Geometry: final body of the model. Coordinates: model frame, mm. A direction names the side the tool comes from. Give positions to 0.01 mm unless a question says otherwise; leave off trailing zeros. Order: outer loops, then holes, each group sorted by start corner. A loop starts at its lowest first (then second) coordinate and runs counter-clockwise, first axis right, second up. Notation, with made-up numbers: (-35.5, 48) -> (17.5, 48) arc R19 ccw to (17.5, 66) -> close; hole circle Ø10 at (83, 24). An arc over 180 degrees is marked (long way). One line per question, with ' | ' between items.
from build123d import *

# Parameters (mm, degrees)
F1_DEPTH  = 2
F3_DEPTH  = 2
F5_DEPTH  = 1
F6_R      = 0.84006
F7_DEPTH  = 1
F8_R      = 0.772284
F9_DEPTH  = 1
F10_W     = 0.575737
F10_H     = 2.122555
F10_W_2   = 0.4
F10_H_2   = 2.778417
F10_H_3   = 2.12387
F10_W_3   = 0.545456
F10_H_4   = 1.760233
F10_W_4   = 0.581819
F10_H_5   = 3.127278
F10_W_5   = 0.472728
F10_H_6   = 4.072734
F10_W_6   = 0.400001
F10_H_7   = 4.181825
F10_W_7   = 0.436365
F10_H_8   = 4.218189
F10_W_8   = 0.509092
F10_H_9   = 3.018187
F10_W_9   = 0.507496
F10_H_10  = 2.769646
F10_W_10  = 0.811112
F11_DEPTH = 0.5


with BuildPart() as f1:
    # F0 (on Top) → F1 (new body)
    with BuildSketch(Plane.XY):
        with BuildLine():
            Line((17.5, 25), (-17.5, 25))
            ThreePointArc((-17.5, 25), (-22.803301, 22.803301), (-25, 17.5))
            Line((-25, 17.5), (-25, -17.5))
            ThreePointArc((-25, -17.5), (-22.803301, -22.803301), (-17.5, -25))
            Line((-17.5, -25), (17.5, -25))
            ThreePointArc((17.5, -25), (22.803301, -22.803301), (25, -17.5))
            Line((25, -17.5), (25, 17.5))
            ThreePointArc((25, 17.5), (22.803301, 22.803301), (17.5, 25))
        make_face()
    extrude(amount=F1_DEPTH)

    # F2 (on face) → F3 (join)
    with BuildSketch(Plane.XY.offset(2)):
        with BuildLine():
            ThreePointArc((-17.337266, -6.77024), (-16.986234, -5.655714), (-16.596286, -4.5542))
            ThreePointArc((-16.596286, -4.5542), (-17.030893, -5.640781), (-17.337266, -6.77024))
        make_face()
        with BuildLine():
            ThreePointArc((0, 13.707489), (-10.053503, 6.171922), (-16.596286, -4.5542))
            ThreePointArc((-16.596286, -4.5542), (-16.986234, -5.655714), (-17.337266, -6.77024))
            ThreePointArc((-17.337266, -6.77024), (-15.200345, -15.343852), (-7.146251, -18.977696))
            ThreePointArc((-7.146251, -18.977696), (2.212472, -19.631089), (11.51198, -18.393445))
            ThreePointArc((11.51198, -18.393445), (18.229392, -13.509449), (18.713062, -5.218303))
            ThreePointArc((18.713062, -5.218303), (18.502407, -4.757976), (18.285647, -4.300492))
            ThreePointArc((18.285647, -4.300492), (10.706603, 6.29139), (0, 13.707489))
        make_face()
        with BuildLine():
            ThreePointArc((18.713062, -5.218303), (18.511326, -4.753823), (18.285647, -4.300492))
            ThreePointArc((18.285647, -4.300492), (18.502407, -4.757976), (18.713062, -5.218303))
        make_face()
    extrude(amount=F3_DEPTH)

    # F4 (on face) → F5 (cut)
    with BuildSketch(Plane.XY.offset(4)):
        with BuildLine():
            Line((-6.871892, 2.191255), (-9.063148, 2.191255))
            ThreePointArc((-9.063148, 2.191255), (-11.253164, 0.073695), (-9.210455, -2.186298))
            Line((-9.210455, -2.186298), (-8.925119, -2.186904))
            Line((-8.925119, -2.186904), (-6.876542, -2.191251))
            ThreePointArc((-6.876542, -2.191251), (-4.680638, -0.002325), (-6.871892, 2.191255))
        make_face()
        with BuildLine():
            Line((-8.925119, -2.186904), (-9.210455, -2.186298))
            ThreePointArc((-9.210455, -2.186298), (-9.067797, -2.191251), (-8.925119, -2.186904))
        make_face()
        with BuildLine():
            Line((10.128108, 2.191255), (7.936852, 2.191255))
            ThreePointArc((7.936852, 2.191255), (5.746836, 0.073695), (7.789545, -2.186298))
            Line((7.789545, -2.186298), (8.074881, -2.186904))
            Line((8.074881, -2.186904), (10.123458, -2.191251))
            ThreePointArc((10.123458, -2.191251), (12.319362, -0.002325), (10.128108, 2.191255))
        make_face()
        with BuildLine():
            Line((8.074881, -2.186904), (7.789545, -2.186298))
            ThreePointArc((7.789545, -2.186298), (7.932203, -2.191251), (8.074881, -2.186904))
        make_face()
        with BuildLine():
            ThreePointArc((-6.770146, -12.095645), (-6.464266, -11.95017), (-6.153883, -11.814569))
            ThreePointArc((-6.153883, -11.814569), (-6.482713, -11.909726), (-6.770146, -12.095645))
        make_face()
        with BuildLine():
            ThreePointArc((4.085766, -12.978509), (-0.882645, -11.0645), (-6.153883, -11.814569))
            ThreePointArc((-6.153883, -11.814569), (-6.464266, -11.95017), (-6.770146, -12.095645))
            ThreePointArc((-6.770146, -12.095645), (-7.094568, -13.392527), (-5.995244, -14.153211))
            ThreePointArc((-5.995244, -14.153211), (-5.884481, -14.14233), (-5.773655, -14.132122))
            ThreePointArc((-5.773655, -14.132122), (-1.437532, -14.261511), (2.746676, -15.40655))
            ThreePointArc((2.746676, -15.40655), (4.494557, -14.787244), (4.085766, -12.978509))
        make_face()
        with BuildLine():
            ThreePointArc((-5.773655, -14.132122), (-5.884481, -14.14233), (-5.995244, -14.153211))
            ThreePointArc((-5.995244, -14.153211), (-5.883949, -14.147927), (-5.773655, -14.132122))
        make_face()
    extrude(amount=-F5_DEPTH, mode=Mode.SUBTRACT)

    # F6 (on face) → F7 (join)
    with BuildSketch(Plane.XY.offset(3)):
        with Locations((-8.223088, 0)):
            Circle(F6_R)
    extrude(amount=F7_DEPTH)

    # F8 (on face) → F9 (join)
    with BuildSketch(Plane.XY.offset(3)):
        with Locations((9.100624, 0)):
            Circle(F8_R)
    extrude(amount=F9_DEPTH)

    # F10 (on face) → F11 (cut)
    with BuildSketch(Plane.XY.offset(4)):
        with Locations((-10.134581, -3.984638)):
            Rectangle(F10_W, F10_H)
        with Locations((-7.127401, -4.31257)):
            Rectangle(F10_W_2, F10_H_2)
        with Locations((-6.472855, -3.985296)):
            Rectangle(F10_W_2, F10_H_3)
        with Locations((-5.818308, -3.803477)):
            Rectangle(F10_W_3, F10_H_4)
        with Locations((7.317732, -4.503073)):
            Rectangle(F10_W_4, F10_H_5)
        with Locations((8.317734, -4.939437)):
            Rectangle(F10_W_5, F10_H_6)
        with Locations((9.263191, -4.957618)):
            Rectangle(F10_W_6, F10_H_7)
        with Locations((10.154101, -4.939436)):
            Rectangle(F10_W_7, F10_H_8)
        with Locations((11.208649, -4.375799)):
            Rectangle(F10_W_8, F10_H_9)
        with Locations((-9.240523, -4.308184)):
            Rectangle(F10_W_9, F10_H_10)
        with Locations((-8.240381, -4.31257)):
            Rectangle(F10_W_10, F10_H_2)
    extrude(amount=-F11_DEPTH, mode=Mode.SUBTRACT)


solid = f1.part
1) Pull-direction query (X, two-part tool) for faces 5 (the flat face through (8, 0, 3)), 6 (the cylindrical face through (-22.745, 22.861, 0.986)), 7 (the flat face through (25, 0, 1)); classes: +X half, -X half, draft (parallel to the pull), parting line (faces both ways), or undercut.
Check result:
face 5: undercut | face 6: -X half | face 7: +X half
2) Material intervals for probe 1 along Y at (x, z) = (-10, 3.75); probe 2 along X at (y, z) = (-1, 3.65); probe 3 along Z at (x, y) = (-20.5, -14), sorted ascending. Write a range as from..to.
Check result:
probe 1: y = -18.65..-5.05, -2.92..-1.98, 1.98..6.23 | probe 2: x = -15.03..-11.01, -4.92..5.99, 12.08..16.49 | probe 3: z = 0..2
3) Set-up query: faces 1 (the cylindrical face through (11, 6, 3)), 2 (the cylindrical face through (2.081, -19.635, 2.986)), 3 (the flat face through (1, -6, 4)), 4 (the cylindrical face through (-0.808, -11.073, 3.507)). Return all of +Z, -Z, +X, -X, +Y, -Y with unobstructed straight access to the full face (end or side cutting, diameter ignored); none if empty.
Check result:
face 1: +Z, +X, +Y | face 2: +Z, -Y | face 3: +Z, +X, -X, +Y, -Y | face 4: +Z
4) Section C-C on x = -18.5. Return loops of the section in (y, z), plus the area to 3 significant figures.
Check result:
outline: (-24.93, 0) -> (24.93, 0) -> (24.93, 2) -> (-24.93, 2) -> close | area: 99.7 mm^2
5) Contact query for flat-ended pins moving along their axis: pin 1 Ø0.6 at (y, z) = (-4.5, 3.5) entering from +X; pin 2 Ø0.6 at (y, z) = (-4, 4) entering from -X; pin 3 Ø0.6 at (x, z) = (-9, 3.5) entering from -Y. Output: stop coordinate, or through.
Check result:
pin 1: stops at x = 18.53 | pin 2: stops at x = -16.5 | pin 3: stops at y = -18.9
6) Section B-B on z = 0.9. Return loops of the section in (x, y), plus the area to 3 significant figures.
Check result:
outline: (-25, -17.5) arc R7.5 ccw to (-17.5, -25) -> (17.5, -25) arc R7.5 ccw to (25, -17.5) -> (25, 17.5) arc R7.5 ccw to (17.5, 25) -> (-17.5, 25) arc R7.5 ccw to (-25, 17.5) -> close | area: 2,450 mm^2
7) Section A-A on y = 3. Return loops of the section in (x, z).
Check result:
outline: (-25, 0) -> (25, 0) -> (25, 2) -> (13.68, 2) -> (13.68, 4) -> (-12.6, 4) -> (-12.6, 2) -> (-25, 2) -> close
